Check sheet for the modelled part. Datum: model origin and axes. Units: mm. Face numbers are marked on the shaded views. A direction names the side the tool comes from. Give positions to 0.01 mm unless a question says otherwise; leave off trailing zeros. Loops run counter-clockwise (first coordinate to the right, second up) from the corner with the lowest first, then second, coordinate; pieces in that order, holes last. Notation, with made-up numbers: (36.25, 44) - (59.25, 44) arc R27 ccw to (59.25, 81) - close; hole circle Ø11 at (87.25, 62.5). An arc over 180 degrees is marked (long way). Answer in a Markdown table with one row per item. Add a question column.
(1) Go/stop test with flat-tipped pins: P1, Ø1.5, axis at x = 6.5, z = -6.5, coming from the -Y side; P2, Ø1.2, axis at y = 2, z = -7, coming from the -X side; P3, Ø5, axis at x = 4.5, z = -7, coming from the +Y side; P4, Ø1.5, axis at x = 2, z = -12, coming from the +Y side. Record where each tip stops, or that it passes through.
(2) Set-up check for the marked faces 1, 2 and 3: record each of +Z, -Z, +X, -X, +Y, -Y from which the full face is reachable in a straight line by a thin tool's end or side.
(3) Thickness scan on L1, parallel to Y at x = 3, z = -3.5; L2, parallel to X at y = 3.95, z = -12.25; L3, parallel to Z at x = 8.25, y = 0.8. Record the ranges inside material, lowest first.
(4) Sectioned sample at C-C on y = 3.55. Enter the section's corners in (x, z), then the cut area to 3 significant figures.
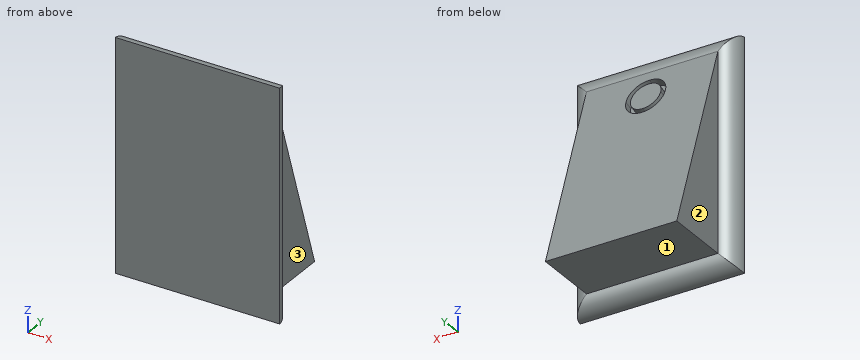
from build123d import *

# Parameters (mm, degrees)
SKETCH1_W           = 10
SKETCH1_H           = 14
BOSS_EXTRUDE1_DEPTH = 1
SKETCH2_W           = 8
SKETCH2_H           = 12
BOSS_EXTRUDE2_DEPTH = 4
CUT_EXTRUDE1_DEPTH  = 8
CUT_EXTRUDE2_DEPTH  = 0.5
FILLET1_R           = 1


with BuildPart() as part:
    # Sketch1 → Boss-Extrude1 (new body)
    with BuildSketch(Plane(origin=(0, 0, 0), x_dir=(1, 0, 0), z_dir=(0, 1, 0))):
        with Locations((5, 7)):
            Rectangle(SKETCH1_W, SKETCH1_H)
    extrude(amount=BOSS_EXTRUDE1_DEPTH)

    # Sketch2 → Boss-Extrude2 (add)
    with BuildSketch(Plane(origin=(0, 1, 0), x_dir=(1, 0, 0), z_dir=(0, 1, 0))):
        with Locations((5, 7)):
            Rectangle(SKETCH2_W, SKETCH2_H)
    extrude(amount=BOSS_EXTRUDE2_DEPTH)

    # Sketch3 → Cut-Extrude1 (cut)
    with BuildSketch(Plane.ZY.offset(-1)):
        Polygon((-13, 5), (-1, 1), (-1, 5), align=None)
    extrude(amount=-CUT_EXTRUDE1_DEPTH, mode=Mode.SUBTRACT)

    # Sketch4 → Cut-Extrude2 (cut)
    with BuildSketch(Plane(origin=(0, 0.6, 0.2), x_dir=(1, 0, 0), z_dir=(0, 0.9486832980505139, 0.3162277660168379))):
        with BuildLine():
            add(Edge.make_bspline(
                [(5.03786558, 4.295135467), (5.08140052, 4.294208466), (5.166761899, 4.292390843), (5.291773338, 4.27296441), (5.411103569, 4.243257872), (5.525209614, 4.202190098), (5.632630111, 4.1471429), (5.73492974, 4.081457329), (5.831828026, 4.003640262), (5.88990606, 3.943444014), (5.919386013, 3.912888873)],
                knots=[0, 0, 0, 0, 1.054011418, 2.066658804, 3.057071809, 4.030435133, 4.997543892, 5.974964718, 6.972108034, 8, 8, 8, 8], degree=3))
            add(Edge.make_bspline(
                [(5.919386013, 3.912888873), (5.944769642, 3.883666186), (5.995045659, 3.825786351), (6.059512418, 3.73193733), (6.115049119, 3.634745954), (6.159556233, 3.532921593), (6.194649076, 3.427353141), (6.219564387, 3.317677745), (6.23438432, 3.204137616), (6.236382726, 3.127026992), (6.237394827, 3.087974009)],
                knots=[0, 0, 0, 0, 1.025258237, 2.030674902, 3.01204498, 3.988269485, 4.97094183, 5.956517959, 6.965070386, 8, 8, 8, 8], degree=3))
            add(Edge.make_bspline(
                [(6.237394827, 3.087974009), (6.236504614, 3.048694671), (6.234745511, 2.971076867), (6.21810523, 2.856759299), (6.192223459, 2.745911139), (6.155183149, 2.638996467), (6.107686864, 2.535688473), (6.049728883, 2.436438382), (5.980902488, 2.341050376), (5.902884577, 2.250334422), (5.816658946, 2.166726499), (5.723117869, 2.093857283), (5.624099567, 2.031426329), (5.518287382, 1.98113758), (5.40664759, 1.941486638), (5.288939393, 1.913637337), (5.16534565, 1.896799238), (5.080956671, 1.894636997), (5.03786558, 1.893532903)],
                knots=[0, 0, 0, 0, 0.998656419, 1.973391657, 2.932242238, 3.890759089, 4.846373663, 5.82037756, 6.809684879, 7.83454468, 8.860553229, 9.859544525, 10.845671541, 11.83227036, 12.833544569, 13.85385346, 14.904124723, 16, 16, 16, 16], degree=3))
            add(Edge.make_bspline(
                [(5.03786558, 1.893532903), (4.99456337, 1.894640703), (4.909753804, 1.896810384), (4.785723807, 1.913571919), (4.667804652, 1.941473803), (4.556018709, 1.981267886), (4.449751598, 2.031427936), (4.350159562, 2.09366854), (4.256542495, 2.166748109), (4.170298624, 2.250328567), (4.092285603, 2.341051884), (4.023457946, 2.436437991), (3.965500293, 2.535688575), (3.918003922, 2.63899644), (3.880963635, 2.745911146), (3.855081858, 2.856759298), (3.838441579, 2.971076868), (3.836682476, 3.048694671), (3.835792263, 3.087974009)],
                knots=[0, 0, 0, 0, 1.099876186, 2.154163076, 3.173186993, 4.173200201, 5.163417411, 6.152872554, 7.150605724, 8.17532212, 9.198891216, 10.186952605, 11.159729845, 12.11414092, 13.071450619, 14.029093627, 15.002601286, 16, 16, 16, 16], degree=3))
            add(Edge.make_bspline(
                [(3.835792263, 3.087974009), (3.836811266, 3.126814733), (3.838828716, 3.203712691), (3.853633749, 3.317039381), (3.878451869, 3.426529156), (3.913586778, 3.531690123), (3.95850413, 3.633068269), (4.013260441, 3.730499794), (4.078384801, 3.823924442), (4.128460857, 3.881729471), (4.153801077, 3.91098082)],
                knots=[0, 0, 0, 0, 1.031353054, 2.041901799, 3.029428768, 4.008703097, 4.981709435, 5.96992636, 6.972712378, 8, 8, 8, 8], degree=3))
            add(Edge.make_bspline(
                [(4.153801077, 3.91098082), (4.183236584, 3.941800943), (4.241126689, 4.002414139), (4.338507321, 4.080004357), (4.440555287, 4.147056796), (4.549162899, 4.20101022), (4.663175206, 4.243499447), (4.783116947, 4.273041021), (4.908552593, 4.29232085), (4.994331678, 4.294187911), (5.03786558, 4.295135467)],
                knots=[0, 0, 0, 0, 1.027980169, 2.021703884, 2.998553061, 3.971491411, 4.943284454, 5.930300938, 6.949603206, 8, 8, 8, 8], degree=3))
        make_face()
        with BuildLine():
            add(Edge.make_bspline(
                [(5.036593545, 4.01019957), (5.005807283, 4.009324547), (4.945029502, 4.007597091), (4.85556745, 3.99445812), (4.769443168, 3.973641456), (4.686493259, 3.944064919), (4.606997453, 3.905875204), (4.530879638, 3.858968334), (4.457915924, 3.803965581), (4.389533624, 3.740953014), (4.326775384, 3.672119926), (4.271913219, 3.598778915), (4.225263301, 3.522119587), (4.186401157, 3.442062224), (4.157456779, 3.357795534), (4.136435537, 3.270273819), (4.123308962, 3.179318762), (4.121597747, 3.117486981), (4.12072816, 3.086065956)],
                knots=[0, 0, 0, 0, 1.021534396, 2.016698045, 2.994645724, 3.958388632, 4.93408049, 5.916473867, 6.921342795, 7.962252576, 8.998418191, 10.008913653, 10.997312074, 11.973003931, 12.956656626, 13.948281152, 14.957379055, 16, 16, 16, 16], degree=3))
            add(Edge.make_bspline(
                [(4.12072816, 3.086065956), (4.122185779, 3.045469474), (4.125078879, 2.964893049), (4.148605843, 2.846228674), (4.187963397, 2.732307994), (4.24111043, 2.623798843), (4.307700357, 2.523403277), (4.386156481, 2.433894145), (4.475636781, 2.356618444), (4.575074606, 2.29250082), (4.68243888, 2.241555899), (4.796064257, 2.205452542), (4.91457403, 2.181983221), (4.995564407, 2.179650527), (5.036593545, 2.178468801)],
                knots=[0, 0, 0, 0, 1.016792936, 2.018143844, 3.017858371, 4.030088057, 5.03801393, 6.028138512, 7.003788237, 7.991172063, 8.984598303, 9.972568034, 10.972917682, 12, 12, 12, 12], degree=3))
            add(Edge.make_bspline(
                [(5.036593545, 2.178468801), (5.077620322, 2.179657412), (5.158606041, 2.182003698), (5.276951152, 2.205334341), (5.390265969, 2.241714091), (5.497518728, 2.292443524), (5.596911289, 2.356861929), (5.687035135, 2.433457785), (5.764821375, 2.52364035), (5.831345431, 2.623931823), (5.885362834, 2.732139771), (5.924536167, 2.846249699), (5.948119691, 2.964887694), (5.951005157, 3.04546768), (5.952458929, 3.086065956)],
                knots=[0, 0, 0, 0, 1.02726834, 2.027799167, 3.010890988, 4.004497153, 4.992059811, 5.971914811, 6.958719428, 7.966827853, 8.981595046, 9.981490638, 10.983022906, 12, 12, 12, 12], degree=3))
            add(Edge.make_bspline(
                [(5.952458929, 3.086065956), (5.951589641, 3.117487169), (5.949879016, 3.179319319), (5.936748155, 3.270271688), (5.915742773, 3.357803351), (5.886739949, 3.442033382), (5.848046665, 3.522326868), (5.800497145, 3.598553835), (5.745859001, 3.672373988), (5.68234347, 3.740730505), (5.614032548, 3.803990145), (5.541039264, 3.858989662), (5.465034319, 3.905669053), (5.385769462, 3.944391571), (5.302808918, 3.973372372), (5.216805308, 3.994578317), (5.127724959, 4.007541566), (5.06716497, 4.009307902), (5.036593545, 4.01019957)],
                knots=[0, 0, 0, 0, 1.042956736, 2.052379634, 3.044323526, 4.02829302, 5.004299113, 5.996692471, 7.007513377, 8.048758398, 9.090003419, 10.095195979, 11.07790575, 12.047570684, 13.018257071, 13.989683339, 14.985167495, 16, 16, 16, 16], degree=3))
        make_face(mode=Mode.SUBTRACT)
    extrude(amount=-CUT_EXTRUDE2_DEPTH, mode=Mode.SUBTRACT)

    # Fillet1
    fillet1_edges = [part.edges().sort_by_distance(p)[0] for p in [
        (5, 1, -14),
        (10, 1, -7),
        (5, 1, 0),
        (0, 1, -7),
    ]]
    fillet(fillet1_edges, radius=FILLET1_R - 0.0001)  # a hair under: the kernel refuses the full size


solid = part.part
Reply:
| question | item | result |
|---|---|---|
| 1 | P1 | y = 0 |
| 1 | P2 | x = 1 |
| 1 | P3 | y = 3.83 |
| 1 | P4 | y = 4.92 |
| 2 | face 1 | -Z, +X, -X, +Y |
| 2 | face 2 | +Z, -Z, -X, +Y |
| 2 | face 3 | +Z, -Z, +X, +Y |
| 3 | L1 | 0 to 1.83 |
| 3 | L2 | 1 to 9 |
| 3 | L3 | -13.6 to -0.4 |
| 4 | outline | (1, -13) - (9, -13) - (9, -8.65) - (1, -8.65) - close |
| 4 | area | 34.8 mm^2 |
